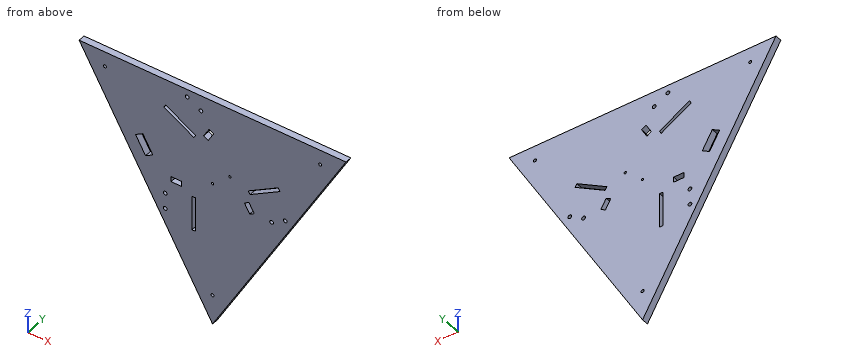
```python
from build123d import *

# Parameters (mm, degrees)
BOSS_EXTRUDE1_DEPTH = 6.35
SKETCH2_W           = 3.302
SKETCH2_H           = 33.02
SKETCH2_R           = 1.778
CUT_EXTRUDE1_DEPTH  = 195.099602868
SKETCH3_R           = 1.4224
SKETCH3_W           = 10
SKETCH3_H           = 5
CUT_EXTRUDE2_DEPTH  = 195.099602868
SKETCH4_R           = 1.0922
CUT_EXTRUDE3_DEPTH  = 195.099602868


with BuildPart() as part:
    # Sketch1 → Boss-Extrude1 (new body)
    with BuildSketch(Plane(origin=(0, 0, 0), x_dir=(1, 0, 0), z_dir=(0, 1, 0))):
        Polygon((0, 146.646968374), (-127, -73.323484187), (127, -73.323484187), align=None)
    extrude(amount=BOSS_EXTRUDE1_DEPTH)

    # Sketch2 → Cut-Extrude1 (cut, through all)
    with BuildSketch(Plane(origin=(0, 6.35, 0), x_dir=(1, 0, 0), z_dir=(0, 1, 0))):
        with Locations((-17.907, 46.362701567)):
            Rectangle(SKETCH2_W, SKETCH2_H)
        Polygon((-16.074197928, -31.864075631), (-17.725197928, -29.004459747), (-46.321356761, -45.514459747), (-44.670356761, -48.374075631), align=None)
        with Locations(Location((-11.086716778, -58.463540546, 0), (0, 0, 270))):
            Circle(SKETCH2_R)
        with Locations(Location((-24.128284992, -65.993093465, 0), (0, 0, 270))):
            Circle(SKETCH2_R)
        Polygon((64.228356761, -14.498625936), (35.632197928, 2.011374064), (33.981197928, -0.848241819), (62.577356761, -17.358241819), align=None)
        with Locations(Location((56.174269697, 19.630391899, 0), (0, 0, 270))):
            Circle(SKETCH2_R)
        with Locations(Location((69.215837912, 12.100838979, 0), (0, 0, 270))):
            Circle(SKETCH2_R)
        Polygon((-56.873789915, 6.738674622), (-66.373789915, -9.71580805), (-73.301993146, -5.71580805), (-63.801993146, 10.738674622), align=None)
        with Locations(Location((-45.087552919, 53.892254486, 0), (0, 0, 270))):
            Circle(SKETCH2_R)
        with Locations(Location((-45.087552919, 38.833148648, 0), (0, 0, 270))):
            Circle(SKETCH2_R)
    extrude(amount=-CUT_EXTRUDE1_DEPTH, mode=Mode.SUBTRACT)

    # Sketch3 → Cut-Extrude2 (cut, through all)
    with BuildSketch(Plane(origin=(0, 6.35, 0), x_dir=(1, 0, 0), z_dir=(0, 1, 0))):
        with Locations(Location((0, 118.312139176, 0), (0, 0, 270))):
            Circle(SKETCH3_R)
        with Locations(Location((-102.461318102, -59.156069588, 0), (0, 0, 270))):
            Circle(SKETCH3_R)
        with Locations(Location((102.461318102, -59.156069588, 0), (0, 0, 270))):
            Circle(SKETCH3_R)
        with Locations((-34.558, 22.352701567)):
            Rectangle(SKETCH3_W, SKETCH3_H)
        Polygon((0.935056109, -41.324967823), (-4.064943891, -32.664713785), (-8.395070909, -35.164713785), (-3.395070909, -43.824967823), align=None)
        Polygon((35.320943891, 21.472266256), (30.320943891, 12.812012218), (34.651070909, 10.312012218), (39.651070909, 18.972266256), align=None)
    extrude(amount=-CUT_EXTRUDE2_DEPTH, mode=Mode.SUBTRACT)

    # Sketch4 → Cut-Extrude3 (cut, through all)
    with BuildSketch(Plane(origin=(0, 6.35, 0), x_dir=(1, 0, 0), z_dir=(0, 1, 0))):
        with Locations(Location((0, 8.207705491, 0), (0, 0, 270))):
            Circle(SKETCH4_R)
        with Locations(Location((16.51, -6.397294509, 0), (0, 0, 270))):
            Circle(SKETCH4_R)
    extrude(amount=-CUT_EXTRUDE3_DEPTH, mode=Mode.SUBTRACT)


solid = part.part
```
Source: CAD feature listing. Evaluate the final solid. Frame: model axes, mm. Round coordinates to 2 decimals unless told otherwise and drop trailing zeros. Write each loop counter-clockwise with the first axis right and the second up, starting at its lowest first coordinate (ties: lowest second). Pieces come first, ordered by that corner, then holes. Notation, with made-up numbers: M 8.25,-20.5 L 29.25,-20.5 A19 cw 29.25,4.5 Z; hole C 53,78.25 d11. An arc over 180 degrees is marked long. Use CSV: the item, a comma, the result in double quotes. Start each with the question number.
Q1. Cut plane D-D on z = -91. Output: boundary loops of the cut face in (x, y), plus the area to 3 significant figures.
Q2. Cut plane B-B on x = 90. Output: boundary loops of the cut face in (y, z), plus the area to 3 significant figures.
Q3. Line query: line 1 (X direction, y = 0.5, z = 38.5); line 2 (X direction, y = 2, z = 33); line 3 (Z direction, x = -18, y = 1.25). Output: solid intervals per line, ascending. Write a range as from..to.
Q4. Cut plane A-A on z = -44.5. Output: boundary loops of the cut face in (x, y), plus the area to 3 significant figures.
Q5. Cut plane C-C on y = 2.25. Count the separate pieces of the cut face and the enclosed holes in it, plus the area to 3 significant figures.
Q6. First-contact query: P1, Ø2.5, axis at y = 2.5, z = -23, coming from the -X side; P2, Ø1.5, axis at y = 4.5, z = -33, coming from the -X side; P3, Ø2.5, axis at x = -102.46, z = 59.16, coming from the -Y side; P4, Ø1.5, axis at x = -94.5, y = 3.5, coming from the -Z side. Flat tips, straight axial feed; report the tip coordinate or a pass-through.
Results found:
1,outline,"M -32.13,0 L 32.13,0 L 32.13,6.35 L -32.13,6.35 Z"
1,area,"408 mm^2"
2,outline,"M 0,9.24 L 6.35,9.24 L 6.35,73.32 L 0,73.32 Z"
2,area,"407 mm^2"
3,line 1,"-106.89..-34.17, -27.57..-6.47, -0.7..106.89"
3,line 2,"-103.72..-24.65, -18.04..-4.65, -3.87..103.72"
3,line 3,"-115.47..-62.87, -29.85..29.16, 32.98..73.32"
4,outline,"M -58.97,0 L -19.56,0 L -19.56,6.35 L -58.97,6.35 Z; M -16.26,0 L 58.97,0 L 58.97,6.35 L -16.26,6.35 Z"
4,area,"728 mm^2"
5,separate pieces,"1"
5,enclosed holes,"18"
5,area,"27,200 mm^2"
6,P1,"x = -72.11"
6,P2,"x = -66.05"
6,P3,"through"
6,P4,"z = 15.73"
